```python
from build123d import *

# Parameters (mm, degrees)
SKETCH1_W           = 6.35
SKETCH1_H           = 12.7
BOSS_EXTRUDE1_DEPTH = 13.208
SKETCH2_W           = 6.35
SKETCH2_H           = 12.7
BOSS_EXTRUDE2_DEPTH = 5.08
SKETCH3_R           = 6.35
BOSS_EXTRUDE3_DEPTH = 6.35
SKETCH4_R           = 1.5875
CUT_EXTRUDE1_DEPTH  = 13.208
MOVE_FACE1_BY       = 0.508


with BuildPart() as part:
    # Sketch1 → Boss-Extrude1 (new body)
    with BuildSketch(Plane.XY):
        Rectangle(SKETCH1_W, SKETCH1_H)
    extrude(amount=BOSS_EXTRUDE1_DEPTH)

    # Sketch2 → Boss-Extrude2 (add)
    with BuildSketch(Plane.ZY.offset(3.175)):
        with Locations((10.033, 0)):
            Rectangle(SKETCH2_W, SKETCH2_H)
    extrude(amount=BOSS_EXTRUDE2_DEPTH)

    # Sketch3 → Boss-Extrude3 (add)
    with BuildSketch(Plane.XY.offset(13.208)):
        with Locations((-8.255, 0)):
            Circle(SKETCH3_R)
    extrude(amount=-BOSS_EXTRUDE3_DEPTH)

    # Sketch4 → Cut-Extrude1 (cut)
    with BuildSketch(Plane(origin=(0, 0, 0), x_dir=(-1, 0, 0), z_dir=(0, 0, -1))):
        with Locations((0, 3.175)):
            Circle(SKETCH4_R)
        with Locations((0, -3.175)):
            Circle(SKETCH4_R)
    extrude(amount=-CUT_EXTRUDE1_DEPTH, mode=Mode.SUBTRACT)

    # Move Face1: a face moved inward by 0.508
    extrude(part.faces().sort_by_distance((-5.513545594, 0, 13.208))[0], amount=MOVE_FACE1_BY, dir=(0, 0, -1), mode=Mode.SUBTRACT)


solid = part.part
```
The model under review builds one solid part; all positions refer to its coordinate system, in mm. A direction names the side the tool comes from. Give positions to 0.01 mm unless a question says otherwise; leave off trailing zeros. Write each loop counter-clockwise with the first axis right and the second up, starting at its lowest first coordinate (ties: lowest second). Pieces come first, ordered by that corner, then holes. Notation, with made-up numbers: (85, 12.25) -> (134, 12.25) arc R30 cw to (134, 45.25) -> close; hole circle Ø7 at (6, 36). An arc over 180 degrees is marked (long way). Put each result on its own line as item: value.
(1) We need section C-C, the plane z = 6. State how many separate pieces and enclosed holes the cut face has, and give its area (3 significant figures).
Results are:
separate pieces: 1
enclosed holes: 2
area: 64.8 mm²
(2) To check wall thickness, follow probe 1 along Y at (x, z) = (0, 7.25); probe 2 along Y at (x, z) = (0.25, 9.75); probe 3 along Z at (x, y) = (-5.25, -0.5). State the ranges of each line that lie inside material, in increasing order. Write a range as from..to.
Results are:
probe 1: -6.35..-4.76, -1.59..1.59, 4.76..6.35
probe 2: -6.35..-4.74, -1.61..1.61, 4.74..6.35
probe 3: 6.86..12.7
(3) Tool access review of faces 1 (the flat face through (-3.175, 0, 3)), 2 (the flat face through (0, 0, 0)): name each direction out of +Z, -Z, +X, -X, +Y, -Y from which nothing blocks a thin tool from reaching the whole face with its end or side.
Results are:
face 1: -Z, -X, +Y, -Y
face 2: -Z, +X, -X, +Y, -Y
(4) We need section D-D, the plane y = 0. Give the boundary of the cut face in (x, z) (3 decimals), and give its area (3 significant figures).
Results are:
outline: (-14.605, 6.858) -> (-3.175, 6.858) -> (-3.175, 0) -> (3.175, 0) -> (3.175, 12.7) -> (-14.605, 12.7) -> close
area: 147 mm²
(5) The part is to be moulded in two halves that separate along Y. For faces 3 (the flat face through (3.175, 0, 6)), 4 (the cylindrical face through (-0.853, 4.514, 6.261)), 5 (the cylindrical face through (-14.603, 0.14, 9.82)), say which applies: pulls with the +Y half, pulls with the -Y half, needs draft (parallel to the pull), parting line crosses it, or undercut.
Results are:
face 3: needs draft
face 4: undercut
face 5: parting line crosses it
(6) For pin 1 Ø1.5 at (x, y) = (-8, 4.5) entering from -Z; pin 2 Ø5.5 at (y, z) = (-1.5, 2.5) entering from -X (3 decimals); pin 3 Ø4 at (x, y) = (0, 3.175) entering from +Z, all flat-tipped, find the tip position at first contact; note any pin that passes through.
Results are:
pin 1: z = 6.86
pin 2: x = -3.175
pin 3: z = 12.7
(7) We need section A-A, the plane x = 0. Give the boundary of the cut face in (y, z).
Results are:
outline: (-6.35, 0) -> (-4.76, 0) -> (-4.76, 12.7) -> (-6.35, 12.7) -> close; (-1.59, 0) -> (1.59, 0) -> (1.59, 12.7) -> (-1.59, 12.7) -> close; (4.76, 0) -> (6.35, 0) -> (6.35, 12.7) -> (4.76, 12.7) -> close
(8) We need section B-B, the plane y = -3.75. Give the boundary of the cut face in (x, z) (3 decimals), and give its area (3 significant figures).
Results are:
outline: (-13.379, 6.858) -> (-3.175, 6.858) -> (-3.175, 0) -> (-1.48, 0) -> (-1.48, 12.7) -> (-13.379, 12.7) -> close; (1.48, 0) -> (3.175, 0) -> (3.175, 12.7) -> (1.48, 12.7) -> close
area: 103 mm²
